The listing builds one solid part. Answer for the finished solid, in the listing's coordinates (mm). A direction names the side the tool comes from. Round coordinates to 2 decimals unless told otherwise and drop trailing zeros. Order: outer loops, then holes, each group sorted by start corner. A loop starts at its lowest first (then second) coordinate and runs counter-clockwise, first axis right, second up. Notation, with made-up numbers: M -39.75,19.5 L -34.75,19.5 A28 cw -34.75,44.5 Z; hole C 26,9 d5. An arc over 180 degrees is marked long. Write item = value, one per line. Start each with the question number.
(1) A cutting plane is placed at D-D, the plane x = 9.25. Determine the outline of the cut face in (y, z).
(2) A cutting plane is placed at B-B, the plane z = 16. Determine the outline of the cut face in (x, y), and give its area (3 significant figures).
(3) A cutting plane is placed at C-C, the plane z = 26. Determine the outline of the cut face in (x, y).
(4) Each of these flat-tipped pins is pushed along its axis until it touches: pin 1 (5.5 mm diameter, centred on x = 1.5, y = 6, fed in from +Z); pin 2 (8 mm diameter, centred on x = 1, z = 39.5, fed in from -Y); pin 3 (2 mm diameter, centred on x = 1, y = -6.5, fed in from +Z). Where does it stop, or does it pass through?
(5) For a pull along Z with two mould halves and no side action, classify faces 1 (the face through (11.5, -0.1, 1)), 2 (the face through (-9, -2.65, 33)), 3 (the face through (-0.049, 9.715, 18.199)), 4 (the face through (9, -2.65, 33)) as released by +Z, released by -Z, zero draft, split by the parting line, or undercut.
(6) Straight lines are drawn through the part: probe 1 along X at (y, z) = (0.5, 41); probe 2 along X at (y, z) = (-0.5, 15); probe 3 along Z at (x, y) = (-2, -6.5). For each, find the intervals that lie inside material, in ascending order. Write a range as from..to.
(7) Which of the six approach directions +Z, -Z, +X, -X, +Y, -Y give full straight-line access (tool end or side, diameter ignored) to faces 5 (the face through (-0.049, -9.699, 18.215)), 6 (the face through (5.64, 0.13, 19.4)), 7 (the face through (9.458, 1.306, 30.194)), 8 (the face through (6.801, 9.715, 30.452)), 9 (the face through (-3.26, 1.85, 9.18))?
(8) A cutting plane is placed at A-A, the plane x = -1.5. Determine the outline of the cut face in (y, z).
from build123d import *

# Parameters (mm, degrees)
F0_W           = 25
F0_H           = 20
F1_DEPTH       = 45
F6_DEPTH       = 12.501
F6_DEPTH_BACK  = 12.501
F4_W           = 30
F4_H           = 26.5
F7_DEPTH       = 6.5
F7_DEPTH_BACK  = 6.5
F8_R           = 3
F9_SIZE        = 2
F10_R          = 1
F11_DEPTH      = 12.5010001
F11_DEPTH_BACK = 12.5010001
F12_DEPTH      = 25


with BuildPart() as f1:
    # F0 (on Top) → F1 (new body)
    with BuildSketch(Plane.XY):
        Rectangle(F0_W, F0_H)
    extrude(amount=F1_DEPTH)

    # F3 (on Right) → F6 (cut, two sides)
    with BuildSketch(Plane.YZ) as f6_sk:
        with BuildLine():
            Line((12.4710435048, 32.5), (12.5, 32.5))
            ThreePointArc((12.5, 32.5), (12.4927587788, 32.9254152033), (12.4710435048, 33.3503375224))
            Line((12.4710435048, 33.3503375224), (12.4710435048, 32.5))
        make_face()
        with BuildLine():
            ThreePointArc((-12.5, 32.5), (-0.4254152033, 44.9927587788), (12.4710435048, 33.3503375224))
            Line((12.4710435048, 33.3503375224), (12.4710435048, 47.7809855342))
            Line((12.4710435048, 47.7809855342), (-12.574961409, 47.7809855342))
            Line((-12.574961409, 47.7809855342), (-12.574961409, 32.5))
            Line((-12.574961409, 32.5), (-12.5, 32.5))
        make_face()
    extrude(amount=-F6_DEPTH, mode=Mode.SUBTRACT)
    extrude(f6_sk.sketch, amount=F6_DEPTH_BACK, mode=Mode.SUBTRACT)

    # F4 (on Right) → F7 (cut, two sides)
    with BuildSketch(Plane.YZ) as f7_sk:
        with Locations((0.1584350094, 31.75)):
            Rectangle(F4_W, F4_H)
    extrude(amount=F7_DEPTH, mode=Mode.SUBTRACT)
    extrude(f7_sk.sketch, amount=-F7_DEPTH_BACK, mode=Mode.SUBTRACT)

    # F8
    f8_edges = [f1.edges().sort_by_distance(p)[0] for p in [
        (6.5, 0, 18.5),
        (-6.5, 0, 18.5),
    ]]
    fillet(f8_edges, radius=F8_R)

    # F9
    f9_edges = [f1.edges().sort_by_distance(p)[0] for p in [
        (12.5, 0, 0),
        (0, 10, 0),
        (-12.5, 0, 0),
        (0, -10, 0),
        (-12.5, 10, 20),
        (12.5, 10, 20),
        (-12.5, -10, 20),
        (12.5, -10, 20),
    ]]
    chamfer(f9_edges, length=F9_SIZE)

    # F10
    f10_edges = [f1.edges().sort_by_distance(p)[0] for p in [
        (6.5, 10, 30.75),
        (6.5, 0, 21.5),
        (6.5, 0, 45),
        (6.5, -10, 30.75),
        (-12.5, 0, 45),
        (-11.458371, 9.041629, 41.131278),
        (-11.458371, -9.041629, 41.131278),
        (-8.5, 10, 40),
        (-8.5, -10, 40),
        (-6.5, 0, 45),
        (8.5, 10, 40),
        (11.458371, 9.041629, 41.131278),
        (12.5, 0, 45),
        (8.5, -10, 40),
        (11.458371, -9.041629, 41.131278),
    ]]
    fillet(f10_edges, radius=F10_R)

    # F5 (on Right) → F11 (cut, two sides)
    with BuildSketch(Plane.YZ) as f11_sk:
        Polygon((-2.65, 30.9700217866), (0, 29.4400435733), (2.65, 30.9700217866), (2.65, 34.0299782134), (0, 35.5599564267), (-2.65, 34.0299782134), align=None)
    extrude(amount=-F11_DEPTH, mode=Mode.SUBTRACT)
    extrude(f11_sk.sketch, amount=F11_DEPTH_BACK, mode=Mode.SUBTRACT)

    # F2 (on face) → F12 (cut)
    with BuildSketch(Plane(origin=(0, 0, 0), x_dir=(1, 0, 0), z_dir=(0, 0, -1))):
        Polygon((4.3301270189, 0), (2.1650635095, 3.75), (-2.1650635095, 3.75), (-4.3301270189, 0), (-2.1650635095, -3.75), (2.1650635095, -3.75), align=None)
    extrude(amount=-F12_DEPTH, mode=Mode.SUBTRACT)


solid = f1.part
Reported:
q1.outline = M -10,2 L -8,0 L 8,0 L 10,2 L 10,39.66 A1 ccw 9.78,40.28 A12.5 ccw -9.78,40.28 A1 ccw -10,39.66 Z; hole M -2.65,30.97 L 0,29.44 L 2.65,30.97 L 2.65,34.03 L 0,35.56 L -2.65,34.03 Z
q2.outline = M -12.5,-8 L -10.5,-10 L 10.5,-10 L 12.5,-8 L 12.5,8 L 10.5,10 L -10.5,10 L -12.5,8 Z; hole M -4.33,0 L -2.17,-3.75 L 2.17,-3.75 L 4.33,0 L 2.17,3.75 L -2.17,3.75 Z
q2.area = 443 mm²
q3.outline = M -12.5,-8 L -10.5,-10 L -7.5,-10 A1 ccw -6.5,-9 L -6.5,9 A1 ccw -7.5,10 L -10.5,10 L -12.5,8 Z; M 6.5,-9 A1 ccw 7.5,-10 L 10.5,-10 L 12.5,-8 L 12.5,8 L 10.5,10 L 7.5,10 A1 ccw 6.5,9 Z
q4.pin_1 = 18.6
q4.pin_2 = through
q4.pin_3 = 18.5
q5.face_1 = released by -Z
q5.face_2 = undercut
q5.face_3 = released by +Z
q5.face_4 = undercut
q6.probe_1 = -12.5..-6.5, 6.5..12.5
q6.probe_2 = -12.5..-4.04, 4.04..12.5
q6.probe_3 = 0..18.5
q7.face_5 = +Z, -Y
q7.face_6 = +Z, +Y, -Y
q7.face_7 = +X, -X
q7.face_8 = +Z, +Y
q7.face_9 = +Z, -Z
q8.outline = M -10,2 L -8,0 L -3.75,0 L -3.75,18.5 L -9,18.5 A1 ccw -10,17.5 Z; M 3.75,0 L 8,0 L 10,2 L 10,17.5 A1 ccw 9,18.5 L 3.75,18.5 Z
